from build123d import *

# Parameters (mm, degrees)
IZIM1_R                     = 75
Y_KSEKLIK_EKSTR_ZYON1_DEPTH = 1080
IZIM2_R                     = 8.5
Y_KSEKLIK_EKSTR_ZYON2_DEPTH = 50
IZIM3_R                     = 50
Y_KSEKLIK_EKSTR_ZYON3_DEPTH = 10
IZIM4_R                     = 7.5
KES_EKSTR_ZYON1_DEPTH       = 1135.966959872
DAIRESEL_KAPLAMA1_COUNT     = 20


with BuildPart() as part:
    # izim1 → Y_kseklik-Ekstr_zyon1 (new body)
    with BuildSketch(Plane.XY):
        Circle(IZIM1_R)
    extrude(amount=Y_KSEKLIK_EKSTR_ZYON1_DEPTH)

    # izim2 → Y_kseklik-Ekstr_zyon2 (add)
    with BuildSketch(Plane.XY.offset(1080)):
        Circle(IZIM2_R)
    y_kseklik_ekstr_zyon2 = extrude(amount=Y_KSEKLIK_EKSTR_ZYON2_DEPTH)

    # Aynalama1: Y_kseklik-Ekstr_zyon2 across plane
    add(y_kseklik_ekstr_zyon2.mirror(Plane.XY.offset(540)))

    # izim3 → Y_kseklik-Ekstr_zyon3 (add)
    with BuildSketch(Plane.XY.offset(1080)):
        Circle(IZIM3_R)
    y_kseklik_ekstr_zyon3 = extrude(amount=Y_KSEKLIK_EKSTR_ZYON3_DEPTH)

    # Aynalama2: Y_kseklik-Ekstr_zyon3 across plane
    add(y_kseklik_ekstr_zyon3.mirror(Plane.XY.offset(540)))

    # izim4 → Kes-Ekstr_zyon1 (cut, through all)
    with BuildSketch(Plane.XY.offset(1080)):
        with Locations((0, 75)):
            Circle(IZIM4_R)
    kes_ekstr_zyon1 = extrude(amount=-KES_EKSTR_ZYON1_DEPTH, mode=Mode.SUBTRACT)

    # Dairesel Kaplama1: Kes-Ekstr_zyon1 ×20 about axis
    dairesel_kaplama1_axis = Axis((0, 0, 0), (0, 0, 1))
    for i in range(1, DAIRESEL_KAPLAMA1_COUNT):
        add(kes_ekstr_zyon1.rotate(dairesel_kaplama1_axis, i * 360 / DAIRESEL_KAPLAMA1_COUNT), mode=Mode.SUBTRACT)


solid = part.part
Can you work these out from the model? Positions are in its coordinate system, mm. A direction names the side the tool comes from. Give positions to 0.01 mm unless a question says otherwise; leave off trailing zeros. One line per item, written item: value. Start each with the question number.
1) I'm going to push flat-ended pins straight in: pin 1 (1.5 mm diameter, centred on x = -31.5, y = -50.5, fed in from +Z); pin 2 (8 mm diameter, centred on x = -55.5, z = 547.5, fed in from +Y); pin 3 (8 mm diameter, centred on y = 38.5, z = 197, fed in from -X). Where does each tip first touch, or does it pass through?
2) On a 3-axis mill with a long thin cutter (end or side, diameter ignored), from which of +Z, -Z, +X, -X, +Y, -Y can I reach the whole of each face in a straight line? I mean faces 1 (the face through (47.69, 15.02, 1084.93)), 2 (the face through (47.69, 15.02, -4.93)). Say none if no direction works.
3) If I drill on line 1 (Y direction, x = -65, z = 131); line 2 (X direction, y = 59.5, z = 150); line 3 (Z direction, x = 51.5, y = 26), over which ranges is the centre line in solid material (lowest first)? Write a range as [from, to].
Completed:
1. pin 1: stops at z = 1080
1. pin 2: stops at y = 54.52
1. pin 3: stops at x = -66.59
2. face 1: +Z
2. face 2: -Z
3. line 1: y = [-37.42, -27.2], [-19.15, 19.15], [27.2, 37.42]
3. line 2: x = [-36.68, 36.68]
3. line 3: z = [0, 1080]
